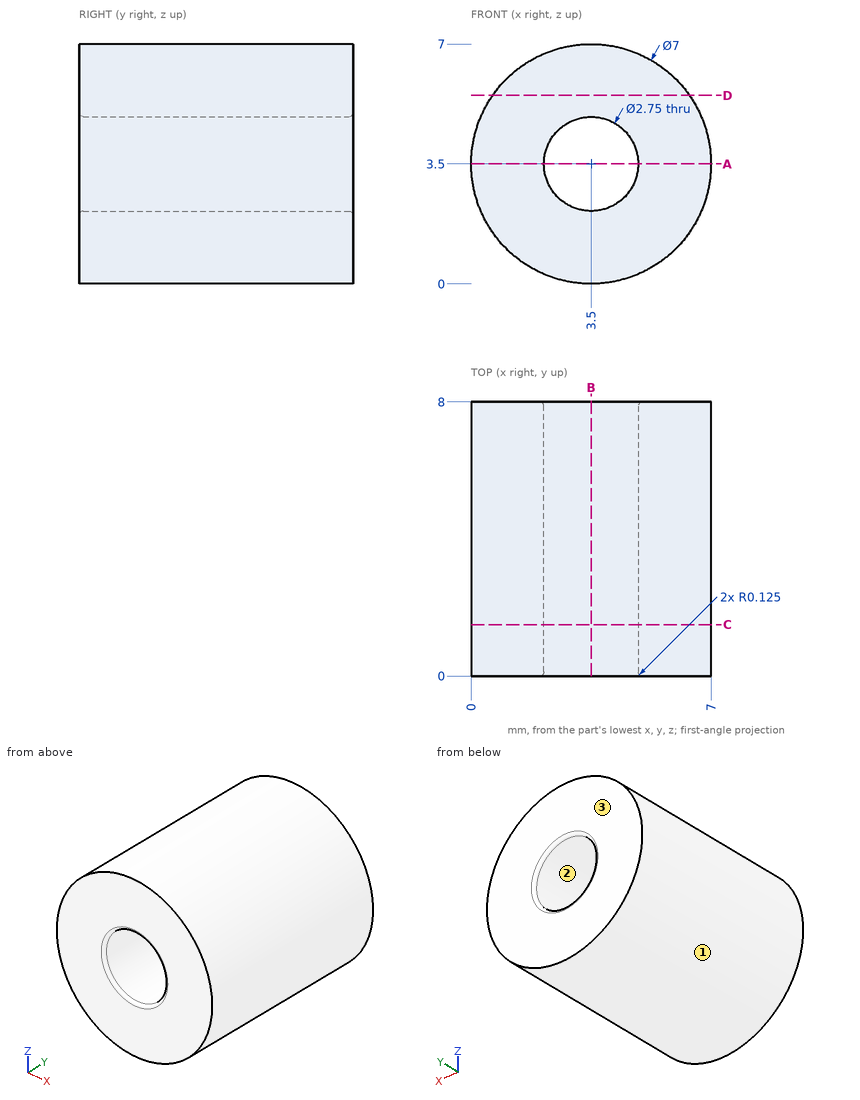
Here's the drawing with two shaded views (mm, measured from the low corner). I have some questions. Round coordinates to 2 decimals unless told otherwise and drop trailing zeros. Loops run counter-clockwise (first coordinate to the right, second up) from the corner with the lowest first, then second, coordinate; pieces in that order, holes last.
Item 1: Will this pin go through, and if not, where does the flat tip stop? pin 1 Ø3 at (x, z) = (5, 1.5) entering from -Y.
Item 2: Suppose I cut it at C-C, the plane y = 1.5. Write out the boundary of the cut face in (x, z) (3 decimals).
Item 3: Suppose I cut it at A-A, the plane z = 3.5. Write out the boundary of the cut face in (x, y) (3 decimals), then the cut area to 3 significant figures.
Item 4: If we mould it in two halves opening along X, with no side actions, what happens to the marked faces 1, 2 and 3? For each: +X half, -X half, draft (parallel to the pull), parting line (faces both ways), or undercut.
Item 5: Please list where these lines run through material, in increasing order: L1, parallel to X at y = 2.5, z = 3.5 (3 decimals); L2, parallel to Z at x = 4.75, y = 4.75.
Item 6: Suppose I cut it at B-B, the plane x = 3.5. Write out the boundary of the cut face in (y, z) (3 decimals).
Item 7: Suppose I cut it at D-D, the plane z = 5.5. Write out the boundary of the cut face in (x, y), then the cut area to 3 significant figures.
Reported:
1. pin 1: stops at y = 0
2. outline: circle Ø7 at (3.5, 3.5); hole circle Ø2.75 at (3.5, 3.5)
3. outline: (0, 0) - (2, 0) arc R0.125 ccw to (2.125, 0.125) - (2.125, 7.875) arc R0.125 ccw to (2, 8) - (0, 8) - close; (4.875, 0.125) arc R0.125 ccw to (5, 0) - (7, 0) - (7, 8) - (5, 8) arc R0.125 ccw to (4.875, 7.875) - close
3. area: 34.0 mm2
4. face 1: parting line
4. face 2: undercut
4. face 3: draft
5. L1: x = 0 to 2.125, 4.875 to 7
5. L2: z = 0.23 to 2.93, 4.07 to 6.77
6. outline: (0, 0) - (8, 0) - (8, 2) arc R0.125 ccw to (7.875, 2.125) - (0.125, 2.125) arc R0.125 ccw to (0, 2) - close; (0, 5) arc R0.125 ccw to (0.125, 4.875) - (7.875, 4.875) arc R0.125 ccw to (8, 5) - (8, 7) - (0, 7) - close
7. outline: (0.63, 0) - (6.37, 0) - (6.37, 8) - (0.63, 8) - close
7. area: 46.0 mm2
